Geometry check sheet. Reference: the model listing, model coordinates, mm. Face numbers are marked on the shaded views. A direction names the side the tool comes from. Give positions to 0.01 mm unless a question says otherwise; leave off trailing zeros. Write each loop counter-clockwise with the first axis right and the second up, starting at its lowest first coordinate (ties: lowest second). Pieces come first, ordered by that corner, then holes. Notation, with made-up numbers: M 74,4 L 96,4 A12 ccw 96,14 Z; hole C 89,3.5 d5. An arc over 180 degrees is marked long. One line per item, written item: value. Start each with the question number.
1. Tool access check on the marked faces 1 and 2. Record the directions out of +Z, -Z, +X, -X, +Y, -Y that give a thin tool (end or side, any length) a straight path to the whole face; none if there is none.
2. Scan lines: line 1 (X direction, y = 7.5, z = 17.5); line 2 (X direction, y = 7.25, z = 29); line 3 (Z direction, x = -18.5, y = 7). Record each from-to range of solid material in increasing order.
3. Cross-section at D-D on z = 8.5. Record the cut outline in (x, y), then the cut area to 3 significant figures.
4. Release check for a two-part mould opening along X. For the marked faces 3, 4 and 5 record: pulls with the +X half, pulls with the -X half, needs draft (parallel to the pull), parting line crosses it, or undercut.
5. Cross-section at C-C on y = -0.75. Record the cut outline in (x, z), then the cut area to 3 significant figures.
6. Gauge pin test, flat ends, axial feed: pin 1 (10 mm diameter, centred on y = -4, z = 17.5, fed in from +X); pin 2 (10 mm diameter, centred on x = -24.5, z = 26, fed in from -Y); pin 3 (4 mm diameter, centred on y = -4, z = 9, fed in from +X); pin 4 (2 mm diameter, centred on x = -23, z = 8.5, fed in from +Y). Record the tip position at first contact, or that the pin passes through.
7. Cross-section at B-B on x = -22. Record the cut outline in (y, z).
8. Cross-section at A-A on y = 6.75. Record the cut outline in (x, z).
from build123d import *

# Parameters (mm, degrees)
F0_R     = 12.5
F1_DEPTH = 10
F2_R     = 12.5
F2_R_2   = 4
F3_DEPTH = 25


with BuildPart() as f1:
    # F0 (on Top) → F1 (new body)
    with BuildSketch(Plane.XY):
        with Locations((-25.3968760371, 4.9218749627)):
            Circle(F0_R)
        Polygon((-17.1604870534, 9.5548433965), (-17.2664131867, 0.1054370842), (-25.5028021704, -4.5275313495), (-33.6332650209, 0.288906529), (-33.5273388876, 9.7383128413), (-25.2909499038, 14.371281275), align=None, mode=Mode.SUBTRACT)
    extrude(amount=F1_DEPTH)

    # F2 (on face) → F3 (join)
    with BuildSketch(Plane.XY.offset(10)):
        with Locations((-25.3968760371, 4.9218749627)):
            Circle(F2_R)
        Polygon((-25.2909499038, 14.371281275), (-17.1604870534, 9.5548433965), (-17.2664131867, 0.1054370842), (-25.5028021704, -4.5275313495), (-33.6332650209, 0.288906529), (-33.5273388876, 9.7383128413), align=None, mode=Mode.SUBTRACT)
        Polygon((-17.2664131867, 0.1054370842), (-17.1604870534, 9.5548433965), (-25.2909499038, 14.371281275), (-33.5273388876, 9.7383128413), (-33.6332650209, 0.288906529), (-25.5028021704, -4.5275313495), align=None)
        with Locations((-25.3968760371, 4.9218749627)):
            Circle(F2_R_2, mode=Mode.SUBTRACT)
    extrude(amount=F3_DEPTH)


solid = f1.part
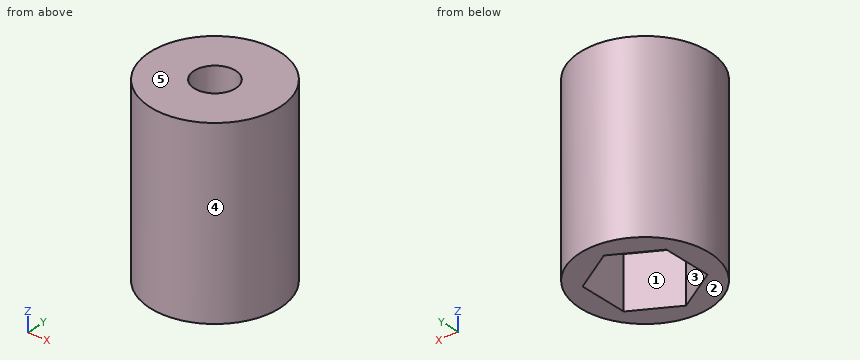
Report:
1. face 1: -Z
1. face 2: -Z, +X, -X, +Y, -Y
2. line 1: x = -37.63 to -28.46, -22.34 to -13.17
2. line 2: x = -37.68 to -28.65, -22.14 to -13.12
2. line 3: z = 10 to 35
3. outline: C -25.4,4.92 d25; hole M -33.63,0.29 L -25.5,-4.53 L -17.27,0.11 L -17.16,9.55 L -25.29,14.37 L -33.53,9.74 Z
3. area: 259 mm^2
4. face 3: undercut
4. face 4: parting line crosses it
4. face 5: needs draft
5. outline: M -36.54,0 L -31.88,0 L -31.88,10 L -18.79,10 L -18.79,0 L -14.26,0 L -14.26,35 L -36.54,35 Z
5. area: 649 mm^2
6. pin 1: stops at x = -13.53
6. pin 2: stops at y = -7.58
6. pin 3: stops at x = -14.99
6. pin 4: stops at y = 17.34
7. outline: M -7.11,0 L -2.56,0 L -2.56,10 L 2.81,10 L 2.81,35 L -7.11,35 Z; M 7.03,10 L 12.42,10 L 12.42,0 L 16.95,0 L 16.95,35 L 7.03,35 Z
8. outline: M -37.76,0 L -33.56,0 L -33.56,10 L -28.95,10 L -28.95,35 L -37.76,35 Z; M -21.84,10 L -17.19,10 L -17.19,0 L -13.03,0 L -13.03,35 L -21.84,35 Z
